```python
from build123d import *

# Parameters (mm, degrees)
F0_R     = 9.8155
F1_DEPTH = 13
F2_R     = 1
F3_T     = -2.5


with BuildPart() as f1:
    # F0 (on Front) → F1 (new body)
    with BuildSketch(Plane.XZ):
        Circle(F0_R)
    extrude(amount=F1_DEPTH)

    # F2
    f2_edges = [f1.edges().sort_by_distance(p)[0] for p in [
        (-9.8155, 0, 0),
    ]]
    fillet(f2_edges, radius=F2_R)

    # F3
    f3_openings = [f1.faces().sort_by_distance(p)[0] for p in [
        (0, -13, 0),
    ]]
    offset(amount=F3_T, openings=f3_openings)


solid = f1.part
```
Geometry check sheet. Reference: the model listing, model coordinates, mm. A direction names the side the tool comes from. Coordinates: 2 decimals unless noted, no trailing zeros. Loops run counter-clockwise (first coordinate to the right, second up) from the corner with the lowest first, then second, coordinate; pieces in that order, holes last. Notation, with made-up numbers: (-32.75, 59) -> (-2.75, 59) arc R23 ccw to (-2.75, 93) -> close; hole circle Ø5 at (35, -3.5). An arc over 180 degrees is marked (long way). Put each result on its own line as item: value.
1) Cross-section at B-B on x = 0. Record the boundary of the cut face in (y, z).
Result set:
outline: (-13, -9.82) -> (-1, -9.82) arc R1 ccw to (0, -8.82) -> (0, 8.82) arc R1 ccw to (-1, 9.82) -> (-13, 9.82) -> (-13, 7.32) -> (-2.5, 7.32) -> (-2.5, -7.32) -> (-13, -7.32) -> close
2) Tool access check on faces 4 (the flat face through (-1.5, -13, 7.32)), 5 (the cylindrical face through (-1.59, -7.68, -7.14)). Record the directions out of +Z, -Z, +X, -X, +Y, -Y that give a thin tool (end or side, any length) a straight path to the whole face; none if there is none.
Result set:
face 4: +Z, -Z, +X, -X, -Y
face 5: -Y
3) Release check for a two-part mould opening along Z. For faces 1 (the flat face through (0, -2.5, 0)), 2 (the flat face through (0, 0, 0)), 3 (the cylindrical face through (9.36, -6.92, 2.95)) record: released by +Z, released by -Z, zero draft, split by the parting line, or undercut.
Result set:
face 1: undercut
face 2: zero draft
face 3: split by the parting line
4) Cross-section at A-A on z = 0. Record the boundary of the cut face in (x, y), plus the area to 3 significant figures.
Result set:
outline: (-9.82, -13) -> (-7.32, -13) -> (-7.32, -2.5) -> (7.32, -2.5) -> (7.32, -13) -> (9.82, -13) -> (9.82, -1) arc R1 ccw to (8.82, 0) -> (-8.82, 0) arc R1 ccw to (-9.82, -1) -> close
area: 101 mm^2
5) Gauge pin test, flat ends, axial feed: pin 1 Ø3 at (y, z) = (-9, 3) entering from -X; pin 2 Ø2 at (y, z) = (-8.5, 5) entering from +X; pin 3 Ø2 at (y, z) = (-2.5, 4) entering from +X. Record the tip position at first contact, or that the pin passes through.
Result set:
pin 1: stops at x = -9.7
pin 2: stops at x = 8.96
pin 3: stops at x = 9.35
6) Cross-section at C-C on y = -3.5. Record the boundary of the cut face in (x, z).
Result set:
outline: circle Ø19.63 at (0, 0); hole circle Ø14.63 at (0, 0)
7) Thickness scan on line 1 (X direction, y = -9.25, z = -0.25); line 2 (Z direction, x = 0, y = -6); line 3 (Y direction, x = -4, z = -1.5). Record the ranges inside material, lowest first.
Result set:
line 1: x = -9.81 to -7.31, 7.31 to 9.81
line 2: z = -9.82 to -7.32, 7.32 to 9.82
line 3: y = -2.5 to 0
